Source: CAD feature listing. Evaluate the final solid. Frame: model axes, mm. A direction names the side the tool comes from. Coordinates: 2 decimals unless noted, no trailing zeros. Order: outer loops, then holes, each group sorted by start corner. A loop starts at its lowest first (then second) coordinate and runs counter-clockwise, first axis right, second up.
```python
from build123d import *

# Parameters (mm, degrees)
F1_DEPTH = 5
F3_DEPTH = 12.001
F5_DEPTH = 5.001
F7_D     = 2.5
F7_DEPTH = 12
F7_TIP   = 0.7510757738
F8_R     = 0.5


with BuildPart() as f1:
    # F0 (on Top) → F1 (new body)
    with BuildSketch(Plane.XY):
        Polygon((0, 17.5), (0, 0), (12, 0), (12, 17.5), (8.5, 21), (3.5, 21), align=None)
    extrude(amount=F1_DEPTH)

    # F2 (on face) → F3 (cut, through all)
    with BuildSketch(Plane.YZ.offset(12)):
        Polygon((0, 3.75), (0, 2.5), (0, 1.25), (2, 2.5), align=None)
    extrude(amount=-F3_DEPTH, mode=Mode.SUBTRACT)

    # F4 (on face) → F5 (cut, through all)
    with BuildSketch(Plane.XY.offset(5)):
        with BuildLine():
            ThreePointArc((9, 10), (3.8786796564, 12.1213203436), (6, 7))
            ThreePointArc((6, 7), (8.1213203436, 7.8786796564), (9, 10))
        make_face()
    extrude(amount=-F5_DEPTH, mode=Mode.SUBTRACT)

    # F7
    with Locations(Plane(origin=(0, 21, 0), x_dir=(-1, 0, 0), z_dir=(0, 1, 0))):
        with Locations((-6, 2.5)):
            Hole(F7_D / 2, depth=F7_DEPTH)
            with Locations((0, 0, -(F7_DEPTH + F7_TIP / 2))):  # 118° drill point
                Cone(0, F7_D / 2, F7_TIP, mode=Mode.SUBTRACT)

    # F8
    f8_edges = [f1.edges().sort_by_distance(p)[0] for p in [
        (1.75, 19.25, 5),
        (3.5, 21, 2.5),
        (1.75, 19.25, 0),
        (6, 21, 5),
        (8.5, 21, 2.5),
        (6, 21, 0),
        (10.25, 19.25, 0),
        (10.25, 19.25, 5),
        (12, 17.5, 2.5),
        (0, 17.5, 2.5),
        (0, 8.75, 5),
        (0, 8.75, 0),
        (12, 8.75, 5),
        (12, 8.75, 0),
        (12, 0, 0.625),
        (6, 0, 1.25),
        (6, 0, 0),
        (12, 0, 4.375),
        (6, 0, 3.75),
        (6, 0, 5),
        (0, 0, 4.375),
        (0, 0, 0.625),
    ]]
    fillet(f8_edges, radius=F8_R)


solid = f1.part
```
1. Pin query (flat end, axial travel): P1, Ø1.5, axis at x = 9.5, z = 0.5, coming from the -Y side. Return the tip coordinate at first contact, or that it passes through.
Findings:
P1: stops at y = 0
2. Ray query, line 1 (Z direction, x = 6, y = 17.75); line 2 (X direction, y = 10, z = 1.25); line 3 (Y direction, x = 6, z = 0.6). Return the intervals inside material, ascending.
Findings:
line 1: z = 0 to 1.25, 3.75 to 5
line 2: x = 0 to 3, 9 to 12
line 3: y = 0 to 7, 13 to 21
3. Access query for faces 4 (the face through (12, 9, 2)), 5 (the face through (6.084, 1.13, 3.044)). Directions: +Z, -Z, +X, -X, +Y, -Y. A direction counts if a zero-diameter tool reaches every point of the face in a straight line with its end or side. Return the directions, or none.
Findings:
face 4: +Z, -Z, +X, +Y, -Y
face 5: +X, -X, -Y
4. Section query A-A on x = 5. Return loops of the section in (y, z) (3 decimals).
Findings:
outline: (0, 0.5) arc R0.5 ccw to (0.5, 0) - (7.172, 0) - (7.172, 5) - (0.5, 5) arc R0.5 ccw to (0, 4.5) - (0, 4.027) arc R0.5 ccw to (0.235, 3.603) - (2, 2.5) - (0.235, 1.397) arc R0.5 ccw to (0, 0.973) - close; (12.828, 0) - (20.5, 0) arc R0.5 ccw to (21, 0.5) - (21, 1.75) - (12.828, 1.75) - close; (12.828, 3.25) - (21, 3.25) - (21, 4.5) arc R0.5 ccw to (20.5, 5) - (12.828, 5) - close
5. Draft query along Z for faces 1 (the face through (4.75, 16.81, 2.55)), 2 (the face through (7, 13, 5)), 3 (the face through (1.834, 19.121, 0.143)). Return one class per face: released by +Z, released by -Z, zero draft, split by the parting line, or undercut.
Findings:
face 1: undercut
face 2: released by +Z
face 3: released by -Z
